Model file for the job. Use its own axes, mm. A direction names the side the tool comes from. Give positions to 0.01 mm unless a question says otherwise; leave off trailing zeros. Write each loop counter-clockwise with the first axis right and the second up, starting at its lowest first coordinate (ties: lowest second). Pieces come first, ordered by that corner, then holes. Notation, with made-up numbers: (19.5, 29) - (53.5, 29) arc R28 ccw to (53.5, 48) - close; hole circle Ø4 at (65.25, -37.5). An arc over 180 degrees is marked (long way). One line per item, written item: value. Start each with the question number.
(1) Cut at B-B, the plane x = -1.5. List the corners of the cut face in (y, z).
(2) Drop flat-ended pins along their axis: P1, Ø4, axis at x = -3, y = 50, coming from the -Z side; P2, Ø5, axis at y = 33.5, z = 4, coming from the +X side. Give the stop position or say it passes through.
(3) Probe L1, parallel to Y at x = -3.5, z = 3.25; L2, parallel to Z at x = -2, y = 12. List the from-to ranges inside material, lowest first.
(4) Cut at A-A, the plane z = 5.5. List the corners of the cut face in (x, y).
(5) 3-axis set-ups, long thin cutter, end or side, ignore diameter. For faces 1 (the face through (0, 0.308, 3)), 2 (the face through (0, -1, 0)): which of +Z, -Z, +X, -X, +Y, -Y reach the whole face in a straight line?
(6) Cut at C-C, the plane y = 4. List the corners of the cut face in (x, z).
(7) Mould opens along Y. For faces 3 (the face through (0, -2.25, 5)), 4 (the face through (-5, 31, 8)), 5 (the face through (0, 61.9, 4)) say: pulls with the +Y half, pulls with the -Y half, needs draft (parallel to the pull), parting line crosses it, or undercut.
Autodesk Inventor part; units mm, degrees
ref_plane "Plano de trabajo1" through (-5, 64.15, -70) normal (0, 1, 0) x (0, 0, 1)
ref_plane "Plano de trabajo2" through (-5, 59.65, 0) normal (0, 0, 1) x (1, 0, 0)
ref_plane "YZ Plane" through (0, 0, 0) normal (1, 0, 0) x (0, 1, 0)
sketch "Boceto1" plane through (0, 0, 0) normal (0, 0, 1) x (1, 0, 0)
  line L0 (-5, 0.3078) -> (-5, -2.25)
  line L1 (5, -2.25) -> (-5, -2.25)
  line L2 (5, 0.3078) -> (5, -2.25)
  line L3 (5, 0.3078) -> (-5, 0.3078)
  point P0 (0, 0)
extrude "Extrusión1" add sketch "Boceto1" along normal blind 10
sketch "Boceto2" plane through (-5, 0.3078, 0) normal (0, 1, 0) x (1, 0, 0)
  line L0 (10, 0) -> (0, 0)
  line L1 (0, 0) -> (0, -10)
  line L2 (10, -10) -> (0, -10)
  line L3 (10, 0) -> (10, -10)
  line L4 (0, 0) -> (0, -10)
  line L5 (0, -10) -> (10, -10)
  line L6 (10, -10) -> (10, -5)
  line L7 (10, -5) -> (0, -5)
  line L8 (0, -5) -> (0, -10)
  line L9 (0, -10) -> (10, -10)
  line L10 (10, -10) -> (10, -7)
  line L11 (10, -7) -> (0, -7)
  line L12 (0, -7) -> (0, -10)
  point P0 (5, 0)
  point P1 (0, -5)
ref_plane "Plano de trabajo1" through (-5, 64.15, -70) normal (0, 1, 0) x (0, 0, 1)
extrude "Extrusión2" add sketch "Boceto2" along normal up to surface (63.8422 mm away) contours L3 L2 L1 L11
sketch "Boceto4" plane through (5, 0.3078, 7) normal (0, 0, -1) x (-1, 0, 0)
  line L0 (10, 63.8422) -> (0, 63.8422)
  line L1 (10, 0) -> (10, 63.8422)
  line L2 (0, 59.3422) -> (0, 63.8422)
  line L3 (10, 63.8422) -> (0, 63.8422)
  line L4 (10, 59.3422) -> (10, 63.8422)
  line L5 (0, 59.3422) -> (10, 59.3422)
  line L6 (10, 61.5922) -> (0, 61.5922)
  point P0 (5, -0.3078)
ref_plane "Plano de trabajo2" through (-5, 59.65, 0) normal (0, 0, 1) x (1, 0, 0)
extrude "Extrusión4" add sketch "Boceto4" along normal up to surface (7 mm away) contours L1 L6 L2 L0
properties part number "Tope trasero"
Answers follow:
1. outline: (-2.25, 0) - (0.31, 0) - (0.31, 7) - (61.9, 7) - (61.9, 0) - (64.15, 0) - (64.15, 10) - (-2.25, 10) - close
2. P1: stops at z = 7
2. P2: passes through
3. L1: y = -2.25 to 0.31, 61.9 to 64.15
3. L2: z = 7 to 10
4. outline: (-5, -2.25) - (5, -2.25) - (5, 0.31) - (-5, 0.31) - close; (-5, 61.9) - (5, 61.9) - (5, 64.15) - (-5, 64.15) - close
5. face 1: -Z, +X, -X
5. face 2: -Z, +X, -X, +Y, -Y
6. outline: (-5, 7) - (5, 7) - (5, 10) - (-5, 10) - close
7. face 3: pulls with the -Y half
7. face 4: needs draft
7. face 5: undercut
